Geometry check sheet. Reference: the model listing, model coordinates, mm. Face numbers are marked on the shaded views. A direction names the side the tool comes from. Coordinates: 2 decimals unless noted, no trailing zeros. Loops run counter-clockwise (first coordinate to the right, second up) from the corner with the lowest first, then second, coordinate; pieces in that order, holes last.
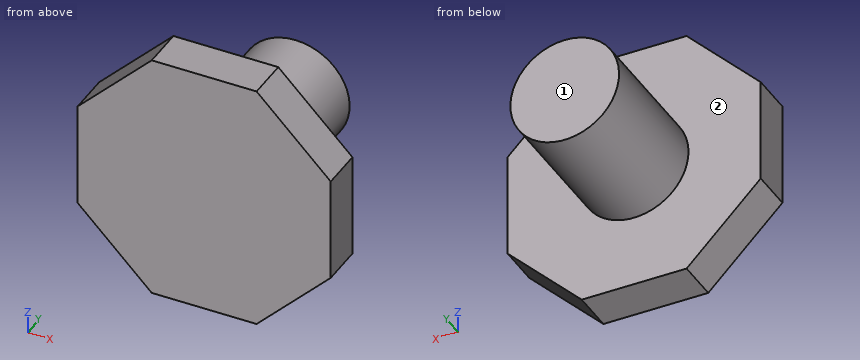
from build123d import *

# Parameters (mm, degrees)
BOSS_EXTRUDE1_DEPTH = 1.5875
SKETCH2_R           = 2.0447
BOSS_EXTRUDE3_DEPTH = 5.08


with BuildPart() as part:
    # Sketch1 → Boss-Extrude1 (new body)
    with BuildSketch(Plane(origin=(0, 0, 0), x_dir=(1, 0, 0), z_dir=(0, 1, 0))):
        Polygon((4.7625, -1.972692091), (4.7625, 1.972692091), (1.972692091, 4.7625), (-1.972692091, 4.7625), (-4.7625, 1.972692091), (-4.7625, -1.972692091), (-1.972692091, -4.7625), (1.972692091, -4.7625), align=None)
    extrude(amount=BOSS_EXTRUDE1_DEPTH)

    # Sketch2 → Boss-Extrude3 (add)
    with BuildSketch(Plane(origin=(0, 1.5875, 0), x_dir=(1, 0, 0), z_dir=(0, 1, 0))):
        with Locations(Location((0, 0, 0), (0, 0, 270))):
            Circle(SKETCH2_R)
    extrude(amount=BOSS_EXTRUDE3_DEPTH)


solid = part.part
(1) Scan lines: L1, parallel to Y at x = -1, z = -2.75; L2, parallel to Z at x = 0.5, y = 6; L3, parallel to X at y = 5.75, z = -1. Record each from-to range of solid material in increasing order.
Findings:
L1: y = 0 to 1.59
L2: z = -1.98 to 1.98
L3: x = -1.78 to 1.78
(2) Sectioned sample at C-C on y = 4. Record the cut outline in (x, z), and give its area (3 significant figures).
Findings:
outline: circle Ø4.09 at (0, 0)
area: 13.1 mm2
(3) Gauge pin test, flat ends, axial feed: pin 1 Ø2 at (x, y) = (1, 3) entering from +Z; pin 2 Ø1 at (y, z) = (2.5, -3.5) entering from -X; pin 3 Ø1.5 at (y, z) = (1.5, 3) entering from +X; pin 4 Ø4 at (y, z) = (5.5, 3.5) entering from +X. Record the tip position at first contact, or that the pin passes through.
Findings:
pin 1: stops at z = 2.04
pin 2: passes through
pin 3: stops at x = 4.49
pin 4: stops at x = 1.39
(4) Access from +Z, -Z, +X, -X, +Y, -Y to the whole of each face (thin tool, end or side, straight path). Record for the marked faces 1 and 2.
Findings:
face 1: +Z, -Z, +X, -X, +Y
face 2: +Y
(5) Sectioned sample at B-B on x = 0. Record the cut outline in (y, z).
Findings:
outline: (0, -4.76) - (1.59, -4.76) - (1.59, -2.04) - (6.67, -2.04) - (6.67, 2.04) - (1.59, 2.04) - (1.59, 4.76) - (0, 4.76) - close
(6) Sectioned sample at D-D on z = -2.75. Record the cut outline in (x, y).
Findings:
outline: (-3.99, 0) - (3.99, 0) - (3.99, 1.59) - (-3.99, 1.59) - close
(7) Sectioned sample at A-A on z = 0. Record the cut outline in (x, y).
Findings:
outline: (-4.76, 0) - (4.76, 0) - (4.76, 1.59) - (2.04, 1.59) - (2.04, 6.67) - (-2.04, 6.67) - (-2.04, 1.59) - (-4.76, 1.59) - close
